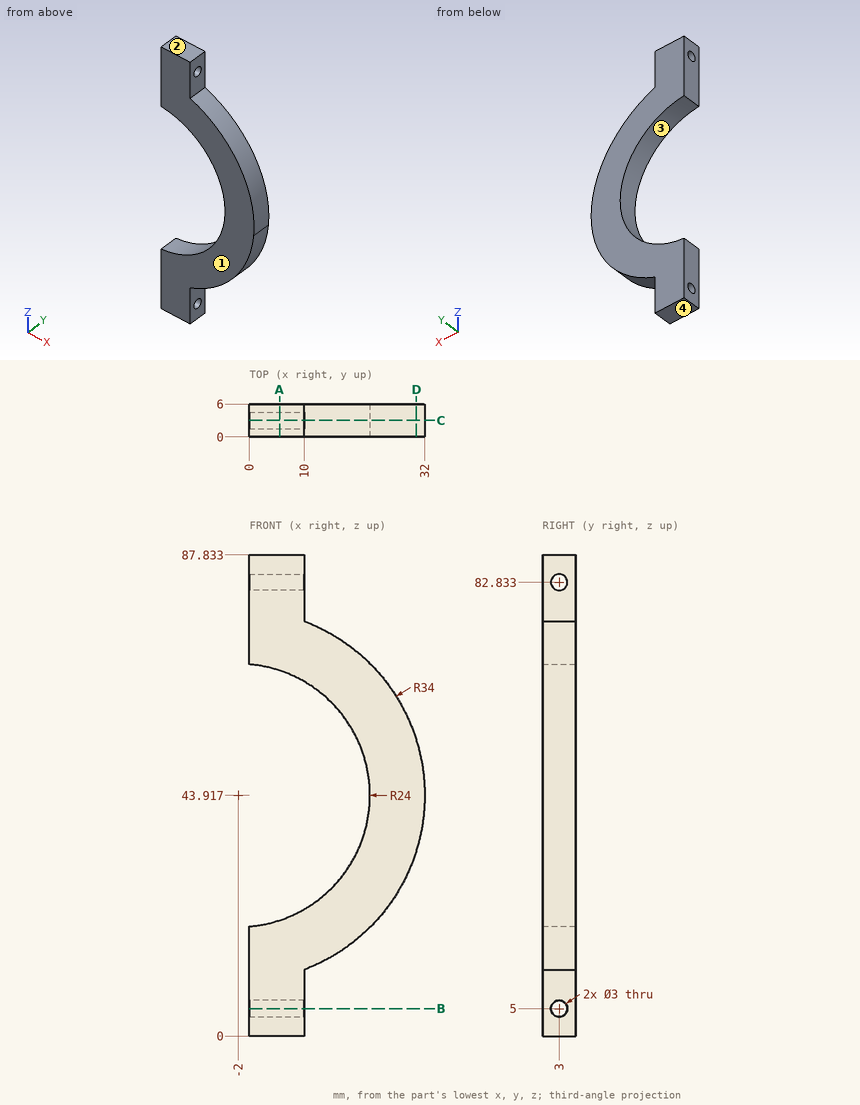
Input: dimensioned drawing with shaded views. Units: mm. Origin: part minimum x, y, z. Round coordinates to 2 decimals unless told otherwise and drop trailing zeros. Loops run counter-clockwise (first coordinate to the right, second up) from the corner with the lowest first, then second, coordinate; pieces in that order, holes last. Notation, with made-up numbers: M -34.75,39 L -22.75,39 A14 ccw -22.75,43 Z; hole C 72,74 d10. An arc over 180 degrees is marked long. Return JSON: item names as keys, results as strings. Group by question number.
1. Pin query (flat end, axial travel): pin 1 (2 mm diameter, centred on x = 13.5, y = 0.5, fed in from -Z); pin 2 (3 mm diameter, centred on y = 2.5, z = 26, fed in from +X) (1 decimal); pin 3 (3.5 mm diameter, centred on y = 3, z = 82.83, fed in from +X). Return the tip coordinate at first contact, or that it passes through.
2. Mould query, pull axis Z, two halves, no side actions, for the marked faces 1, 2, 3 and 4. Classes: released by +Z, released by -Z, zero draft, split by the parting line, or undercut.
3. Material intervals for line 1 along Y through (x, z) = (4, 5); line 2 along Z through (x, y) = (6, 3.4) (1 decimal); line 3 along Z through (x, y) = (6, 3.8) (1 decimal), sorted ascending. Write a range as from..to.
4. Section query D-D on x = 30.5. Output: boundary loops of the cut face in (y, z).
5. Section query B-B on z = 5. Output: boundary loops of the cut face in (x, y), and give its area (3 significant figures).
6. Section query C-C on y = 3. Output: boundary loops of the cut face in (x, z) (1 decimal).
7. Section query A-A on x = 5.5. Output: boundary loops of the cut face in (y, z) (1 decimal).
Checks:
{
 "1": {"pin 1": "stops at z = 13.16", "pin 2": "stops at x = 27.8", "pin 3": "stops at x = 10"},
 "2": {"face 1": "zero draft", "face 2": "released by +Z", "face 3": "undercut", "face 4": "released by -Z"},
 "3": {"line 1": "y = 0..1.5, 4.5..6", "line 2": "z = 0..3.6, 6.4..21.3, 66.5..81.4, 84.3..87.8", "line 3": "z = 0..3.7, 6.3..21.3, 66.5..81.6, 84.1..87.8"},
 "4": {"outline": "M 0,33.93 L 6,33.93 L 6,53.9 L 0,53.9 Z"},
 "5": {"outline": "M 0,0 L 10,0 L 10,1.5 L 0,1.5 Z; M 0,4.5 L 10,4.5 L 10,6 L 0,6 Z", "area": "30.0 mm²"},
 "6": {"outline": "M 0,0 L 10,0 L 10,3.5 L 0,3.5 Z; M 0,6.5 L 10,6.5 L 10,12.1 A34 ccw 10,75.7 L 10,81.3 L 0,81.3 L 0,67.8 A24 cw 0,20 Z; M 0,84.3 L 10,84.3 L 10,87.8 L 0,87.8 Z"},
 "7": {"outline": "M 0,0 L 6,0 L 6,21.1 L 0,21.1 Z; M 0,66.7 L 6,66.7 L 6,87.8 L 0,87.8 Z; hole C 3,5 d3; hole C 3,82.8 d3"}
}
